```python
from build123d import *

# Parameters (mm, degrees)
F0_W          = 19.5
F0_H          = 9.8
F1_DEPTH      = 5
F3_D          = 3.3
F4_R          = 5
F5_R          = 1
F7_DEPTH      = 4.901
F7_DEPTH_BACK = 4.901


with BuildPart() as f1:
    # F0 (on Top) → F1 (new body)
    with BuildSketch(Plane.XY):
        Rectangle(F0_W, F0_H)
    extrude(amount=F1_DEPTH)

    # F3 (through all)
    with Locations(Plane.XY.offset(5)):
        with Locations((0, 0)):
            Hole(F3_D / 2)

    # F4
    f4_edges = [f1.edges().sort_by_distance(p)[0] for p in [
        (-9.75, -4.9, 2.5),
        (9.75, 4.9, 2.5),
    ]]
    fillet(f4_edges, radius=F4_R)

    # F5
    f5_edges = [f1.edges().sort_by_distance(p)[0] for p in [
        (-9.75, 4.9, 2.5),
        (9.75, -4.9, 2.5),
    ]]
    fillet(f5_edges, radius=F5_R)

    # F6 (on Front) → F7 (cut, two sides)
    with BuildSketch(Plane.XZ) as f7_sk:
        Polygon((9.75, 3.1), (5.75, 0), (9.75, 0), align=None)
        Polygon((-9.75, 3.1), (-9.75, 0), (-5.75, 0), align=None)
    extrude(amount=-F7_DEPTH, mode=Mode.SUBTRACT)
    extrude(f7_sk.sketch, amount=F7_DEPTH_BACK, mode=Mode.SUBTRACT)


solid = f1.part
```
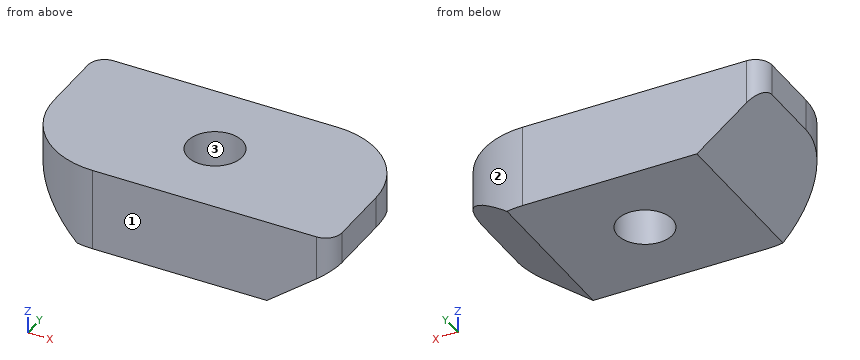
Source: CAD feature listing. Evaluate the final solid. Frame: model axes, mm. Face numbers are marked on the shaded views. Give positions to 0.01 mm unless a question says otherwise; leave off trailing zeros. Loops run counter-clockwise (first coordinate to the right, second up) from the corner with the lowest first, then second, coordinate; pieces in that order, holes last. Notation, with made-up numbers: M 34.25,56 L 77.25,56 A12 ccw 77.25,68 Z; hole C 13,41 d5. An arc over 180 degrees is marked long. Put each result on its own line as item: value.
Q1. Section B-B (y = -0.5). Return the cut outline in (x, z), and give its area (3 significant figures).
Response values:
outline: M -9.71,3.07 L -5.75,0 L -1.57,0 L -1.57,5 L -9.71,5 Z; M 1.57,0 L 5.75,0 L 9.75,3.1 L 9.75,5 L 1.57,5 Z
area: 69.3 mm²
Q2. Mould query, pull axis Y, two halves, no side actions, for the marked faces 1, 2 and 3. Classes: released by +Y, released by -Y, zero draft, split by the parting line, or undercut.
Response values:
face 1: released by -Y
face 2: released by +Y
face 3: undercut
Q3. Section C-C (z = 1.85). Return the cut outline in (x, y), and give its area (3 significant figures).
Response values:
outline: M -8.14,-3.58 A5 ccw -4.75,-4.9 L 8.14,-4.9 L 8.14,3.58 A5 ccw 4.75,4.9 L -8.14,4.9 Z; hole C 0,0 d3.3
area: 148 mm²
Q4. Pin query (flat end, axial travel): P1, Ø1.5, axis at y = 3, z = 2, coming from the -X side; P2, Ø3, axis at x = 2, y = -3, coming from the -Z side; P3, Ø1, axis at y = 1.5, z = 0.5, coming from the -X side. Return the tip coordinate at first contact, or that it passes through.
Response values:
P1: stops at x = -9.3
P2: stops at z = 0
P3: stops at x = -7.04
Q5. Section A-A (x = 0). Return the cut outline in (y, z), and give its area (3 significant figures).
Response values:
outline: M -4.9,0 L -1.65,0 L -1.65,5 L -4.9,5 Z; M 1.65,0 L 4.9,0 L 4.9,5 L 1.65,5 Z
area: 32.5 mm²
Q6. Section D-D (y = 2.25). Return the cut outline in (x, z).
Response values:
outline: M -9.75,3.1 L -5.75,0 L 5.75,0 L 9.16,2.65 L 9.16,5 L -9.75,5 Z
Q7. Line query: probe 1 along Y at (x, z) = (0, 3.55); probe 2 along Y at (x, z) = (0.75, 3.05); probe 3 along X at (y, z) = (-3.5, 0.3). Output: solid intervals per line, ascending. Write a range as [from, to].
Response values:
probe 1: y = [-4.9, -1.65], [1.65, 4.9]
probe 2: y = [-4.9, -1.47], [1.47, 4.9]
probe 3: x = [-6.14, 6.14]
